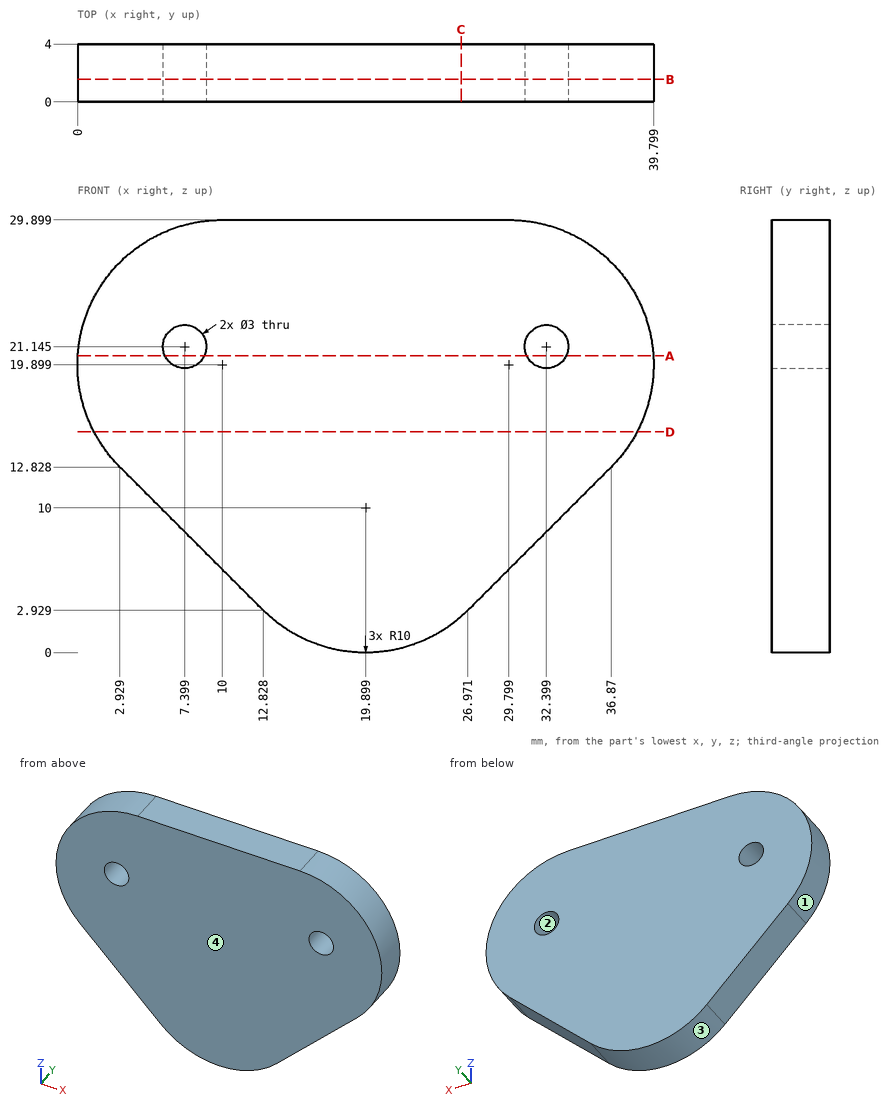
Could you check a few things on this drawing? It's one solid part, dimensions in mm from its lowest x, y, z. Round coordinates to 2 decimals unless told otherwise and drop trailing zeros. Write each loop counter-clockwise with the first axis right and the second up, starting at its lowest first coordinate (ties: lowest second). Pieces come first, ordered by that corner, then holes.
Q1. If we section it at D-D on z = 15.25: Write out the boundary of the cut face in (x, y).
Q2. If we section it at A-A on z = 20.5: Write out the boundary of the cut face in (x, y) (1 decimal).
Q3. Please list where these lines run through material, in increasing order: probe 1 along X at (y, z) = (2.75, 20.5) (1 decimal); probe 2 along Z at (x, y) = (31.5, 1.85) (1 decimal); probe 3 along Z at (x, y) = (33.5, 2.5) (1 decimal).
Q4. If we section it at C-C on x = 26.5: Write out the boundary of the cut face in (y, z), plus the area to 3 significant figures.
Q5. If we mould it in two halves opening along Z, with no side actions, what happens to the marked faces 1, 2, 3 and 4? For each: +Z half, -Z half, draft (parallel to the pull), parting line (faces both ways), or undercut.
Q6. If we section it at B-B on y = 1.55: Write out the boundary of the cut face in (x, z) (1 decimal), plus the area to 3 significant figures.
Q7. Will this pin go through, and if not, where does the flat tip stop? P1, Ø2.5, axis at x = 7.4, z = 21.14, coming from the +Y side.
Answer below:
1. outline: (1.15, 0) - (38.65, 0) - (38.65, 4) - (1.15, 4) - close
2. outline: (0, 0) - (6, 0) - (6, 4) - (0, 4) - close; (8.8, 0) - (31, 0) - (31, 4) - (8.8, 4) - close; (33.8, 0) - (39.8, 0) - (39.8, 4) - (33.8, 4) - close
3. probe 1: x = 0 to 6, 8.8 to 31, 33.8 to 39.8
3. probe 2: z = 7.5 to 19.9, 22.3 to 29.8
3. probe 3: z = 9.5 to 20.1, 22.2 to 29.2
4. outline: (0, 2.49) - (4, 2.49) - (4, 29.9) - (0, 29.9) - close
4. area: 110 mm2
5. face 1: parting line
5. face 2: undercut
5. face 3: -Z half
5. face 4: draft
6. outline: (2.9, 12.8) - (12.8, 2.9) arc R10 ccw to (27, 2.9) - (36.9, 12.8) arc R10 ccw to (29.8, 29.9) - (10, 29.9) arc R10 ccw to start; hole circle Ø3 at (7.4, 21.1); hole circle Ø3 at (32.4, 21.1)
6. area: 876 mm2
7. P1: passes through
